The listing builds one solid part. Answer for the finished solid, in the listing's coordinates (mm). A direction names the side the tool comes from. Give positions to 0.01 mm unless a question says otherwise; leave off trailing zeros. Loops run counter-clockwise (first coordinate to the right, second up) from the corner with the lowest first, then second, coordinate; pieces in that order, holes last. Notation, with made-up numbers: (71.5, 22.5) - (77.5, 22.5) arc R21 ccw to (77.5, 48.5) - close; hole circle Ø6 at (-33.75, -36.75). An arc over 180 degrees is marked (long way). Answer in a Markdown table with one row per item. Add a question column.
```python
from build123d import *

# Parameters (mm, degrees)
F0_W           = 152.4
F0_H           = 152.4
F0_W_2         = 28.2842712475
F0_H_2         = 28.2842712475
F1_DEPTH       = 6.35
F2_D           = 6.6
F2_CBORE_D     = 12
F2_CBORE_DEPTH = 3.5
F3_R           = 50.8
F4_R           = 6
F5_DEPTH       = 1


with BuildPart() as f1:
    # F0 (on Top) → F1 (new body)
    with BuildSketch(Plane.XY):
        Rectangle(F0_W, F0_H)
        with BuildLine():
            ThreePointArc((0, -63.3095), (3.3655, -66.675), (0, -70.0405))
            ThreePointArc((0, -70.0405), (-35.02025, -60.6568522938), (-60.6568522938, -35.02025))
            ThreePointArc((-60.6568522938, -35.02025), (-59.4249937973, -30.4228915036), (-54.8276353009, -31.65475))
            ThreePointArc((-54.8276353009, -31.65475), (-31.65475, -54.8276353009), (0, -63.3095))
        make_face(mode=Mode.SUBTRACT)
        with BuildLine():
            ThreePointArc((-54.8276353009, 31.65475), (-59.4249937973, 30.4228915036), (-60.6568522938, 35.02025))
            ThreePointArc((-60.6568522938, 35.02025), (-35.02025, 60.6568522938), (0, 70.0405))
            ThreePointArc((0, 70.0405), (3.3655, 66.675), (0, 63.3095))
            ThreePointArc((0, 63.3095), (-31.65475, 54.8276353009), (-54.8276353009, 31.65475))
        make_face(mode=Mode.SUBTRACT)
        Rectangle(F0_W_2, F0_H_2, mode=Mode.SUBTRACT)
        with BuildLine():
            ThreePointArc((54.8276353009, 31.65475), (56.0594937973, 36.2521084964), (60.6568522938, 35.02025))
            ThreePointArc((60.6568522938, 35.02025), (70.0405, 0), (60.6568522938, -35.02025))
            ThreePointArc((60.6568522938, -35.02025), (56.0594937973, -36.2521084964), (54.8276353009, -31.65475))
            ThreePointArc((54.8276353009, -31.65475), (63.3095, 0), (54.8276353009, 31.65475))
        make_face(mode=Mode.SUBTRACT)
        Rectangle(F0_W_2, F0_H_2)
    extrude(amount=-F1_DEPTH)

    # F2 (through all)
    with Locations(Plane.XY):
        with Locations((14.1421356237, 14.1421356237), (14.1421356237, -14.1421356237), (-14.1421356237, -14.1421356237), (-14.1421356237, 14.1421356237)):
            CounterBoreHole(F2_D / 2, F2_CBORE_D / 2, F2_CBORE_DEPTH)

    # F3
    f3_edges = [f1.edges().sort_by_distance(p)[0] for p in [
        (76.2, -76.2, -3.175),
        (-76.2, -76.2, -3.175),
        (76.2, 76.2, -3.175),
        (-76.2, 76.2, -3.175),
    ]]
    fillet(f3_edges, radius=F3_R)

    # F4 (on face) → F5 (cut)
    with BuildSketch(Plane(origin=(0, 0, -6.35), x_dir=(1, 0, 0), z_dir=(0, 0, -1))):
        with BuildLine():
            ThreePointArc((-76.2, -25.4), (-61.3210244843, -61.3210244843), (-25.4, -76.2))
            Line((-25.4, -76.2), (25.4, -76.2))
            ThreePointArc((25.4, -76.2), (61.3210244843, -61.3210244843), (76.2, -25.4))
            Line((76.2, -25.4), (76.2, 25.4))
            ThreePointArc((76.2, 25.4), (61.3210244843, 61.3210244843), (25.4, 76.2))
            Line((25.4, 76.2), (-25.4, 76.2))
            ThreePointArc((-25.4, 76.2), (-61.3210244843, 61.3210244843), (-76.2, 25.4))
            Line((-76.2, 25.4), (-76.2, -25.4))
        make_face()
        with BuildLine():
            ThreePointArc((-54.8276353009, -31.65475), (-31.65475, -54.8276353009), (0, -63.3095))
            ThreePointArc((0, -63.3095), (3.3655, -66.675), (0, -70.0405))
            ThreePointArc((0, -70.0405), (-35.02025, -60.6568522938), (-60.6568522938, -35.02025))
            ThreePointArc((-60.6568522938, -35.02025), (-59.4249937973, -30.4228915036), (-54.8276353009, -31.65475))
        make_face(mode=Mode.SUBTRACT)
        with Locations((-14.1421356237, -14.1421356237)):
            Circle(F4_R, mode=Mode.SUBTRACT)
        with Locations((14.1421356237, -14.1421356237)):
            Circle(F4_R, mode=Mode.SUBTRACT)
        with BuildLine():
            ThreePointArc((60.6568522938, -35.02025), (56.0594937973, -36.2521084964), (54.8276353009, -31.65475))
            ThreePointArc((54.8276353009, -31.65475), (63.3095, 0), (54.8276353009, 31.65475))
            ThreePointArc((54.8276353009, 31.65475), (56.0594937973, 36.2521084964), (60.6568522938, 35.02025))
            ThreePointArc((60.6568522938, 35.02025), (70.0405, 0), (60.6568522938, -35.02025))
        make_face(mode=Mode.SUBTRACT)
        with Locations((-14.1421356237, 14.1421356237)):
            Circle(F4_R, mode=Mode.SUBTRACT)
        with BuildLine():
            ThreePointArc((-54.8276353009, 31.65475), (-59.4249937973, 30.4228915036), (-60.6568522938, 35.02025))
            ThreePointArc((-60.6568522938, 35.02025), (-35.02025, 60.6568522938), (0, 70.0405))
            ThreePointArc((0, 70.0405), (3.3655, 66.675), (0, 63.3095))
            ThreePointArc((0, 63.3095), (-31.65475, 54.8276353009), (-54.8276353009, 31.65475))
        make_face(mode=Mode.SUBTRACT)
        with Locations((14.1421356237, 14.1421356237)):
            Circle(F4_R, mode=Mode.SUBTRACT)
    extrude(amount=-F5_DEPTH, mode=Mode.SUBTRACT)


solid = f1.part
```
(1) Given pin 1 Ø4 at (x, y) = (14.14, 14.14) entering from -Z; pin 2 Ø10.5 at (x, y) = (-14.14, -14.14) entering from +Z; pin 3 Ø2 at (x, z) = (59, -4) entering from -Y; pin 4 Ø1.5 at (y, z) = (-36.5, -5.5) entering from +X, each flat-ended and moving along its own axis, determine where each tip first touches the part or whether it passes through.
(2) A cutting plane is placed at C-C on y = 47. Determine the outline of the cut face in (x, z), plus the area to 3 significant figures.
(3) A cutting plane is placed at B-B on z = -1. Determine the outline of the cut face in (x, y) (1 decimal), plus the area to 3 significant figures.
(4) The mould has two halves that part along X. Classify faces 1 (the face through (60.924, -61.714, -2.712)), 2 (the face through (8.148, 13.878, -5.857)), 3 (the face through (-76.2, 0, -3)): pulls with the +X half, pulls with the -X half, needs draft (parallel to the pull), parting line crosses it, or undercut.
(5) A cutting plane is placed at D-D on x = -45. Determine the outline of the cut face in (y, z).
(6) A tool of negligible diameter and unlimited length cuts with its end or side. For faces 4 (the face through (-18.564, 10.087, -5.857)), 5 (the face through (63.308, -0.464, -2.638)), 6 (the face through (8.148, -13.878, -1.726)), from which of +Z, -Z, +X, -X, +Y, -Y can it reach the whole face along a straight path? Write none if from no direction.
(7) A cutting plane is placed at A-A on x = -3. Determine the outline of the cut face in (y, z), plus the area to 3 significant figures.
(8) Find the intervals of material crossed by line 1 along X through (y, z) = (-1, -0.75); line 2 along Y through (x, z) = (-19.5, -4.75); line 3 along Y through (x, z) = (0.5, -3), in increasing order. Write a range as [from, to].
Evaluation:
| question | item | result |
|---|---|---|
| 1 | pin 1 | passes through |
| 1 | pin 2 | stops at z = -3.5 |
| 1 | pin 3 | stops at y = -64.36 |
| 1 | pin 4 | stops at x = 75.13 |
| 2 | outline | (-71.38, -5.35) - (-51.93, -5.35) - (-51.93, 0) - (-71.38, 0) - close; (-42.42, -5.35) - (71.38, -5.35) - (71.38, 0) - (-42.42, 0) - close |
| 2 | area | 713 mm² |
| 3 | outline | (-76.2, -25.4) arc R50.8 ccw to (-25.4, -76.2) - (25.4, -76.2) arc R50.8 ccw to (76.2, -25.4) - (76.2, 25.4) arc R50.8 ccw to (25.4, 76.2) - (-25.4, 76.2) arc R50.8 ccw to (-76.2, 25.4) - close; hole (-60.7, -35) arc R70 ccw to (0, -70) arc R3.4 ccw to (0, -63.3) arc R63.3 cw to (-54.8, -31.7) arc R3.4 ccw to start; hole (-60.7, 35) arc R3.4 ccw to (-54.8, 31.7) arc R63.3 cw to (0, 63.3) arc R3.4 ccw to (0, 70) arc R70 ccw to start; hole circle Ø12 at (-14.1, -14.1); hole circle Ø12 at (-14.1, 14.1); hole circle Ø12 at (14.1, -14.1); hole circle Ø12 at (14.1, 14.1); hole (54.8, -31.7) arc R3.4 ccw to (60.7, -35) arc R70 ccw to (60.7, 35) arc R3.4 ccw to (54.8, 31.7) arc R63.3 cw to start |
| 3 | area | 19,000 mm² |
| 4 | face 1 | pulls with the +X half |
| 4 | face 2 | undercut |
| 4 | face 3 | pulls with the -X half |
| 5 | outline | (-72.27, -5.35) - (-53.67, -5.35) - (-53.67, 0) - (-72.27, 0) - close; (-44.53, -5.35) - (44.53, -5.35) - (44.53, 0) - (-44.53, 0) - close; (53.67, -5.35) - (72.27, -5.35) - (72.27, 0) - (53.67, 0) - close |
| 6 | face 4 | -Z |
| 6 | face 5 | +Z, -Z |
| 6 | face 6 | +Z |
| 7 | outline | (-76.2, -5.35) - (-69.98, -5.35) - (-69.98, 0) - (-76.2, 0) - close; (-63.24, -5.35) - (63.24, -5.35) - (63.24, 0) - (-63.24, 0) - close; (69.98, -5.35) - (76.2, -5.35) - (76.2, 0) - (69.98, 0) - close |
| 7 | area | 743 mm² |
| 8 | line 1 | x = [-76.2, 63.3], [70.03, 76.2] |
| 8 | line 2 | y = [-76.2, -67.27], [-60.23, 60.23], [67.27, 76.2] |
| 8 | line 3 | y = [-76.2, -70], [-63.35, 63.35], [70, 76.2] |
